The model under review builds one solid part; all positions refer to its coordinate system, in mm. A direction names the side the tool comes from. Round coordinates to 2 decimals unless told otherwise and drop trailing zeros. Write each loop counter-clockwise with the first axis right and the second up, starting at its lowest first coordinate (ties: lowest second). Pieces come first, ordered by that corner, then holes. Notation, with made-up numbers: (-30.75, -19.5) -> (17.25, -19.5) arc R21 cw to (17.25, 18.5) -> close; hole circle Ø1 at (22.5, -30.5). An arc over 180 degrees is marked (long way). Return JSON: item names as keys, results as strings. Group by question number.
1. Clearance check with flat-ended pins moving along their axes: P1, Ø4, axis at y = 2.5, z = -16, coming from the -X side; P2, Ø1.4, axis at x = -58, y = 0.5, coming from the -Z side; P3, Ø4, axis at x = 41, y = 1, coming from the +Z side; P4, Ø6, axis at x = 21.5, z = 11, coming from the -Y side. State where each tip first meets the part, or that it passes through.
2. Take a section at B-B, the plane x = 47. Write out the cut boundary in (y, z).
3. Tool access review of faces 4 (the cylindrical face through (-17.124, 0.049, -11.02)), 5 (the cylindrical face through (-46.17, -0.71, -16.59)), 6 (the cylindrical face through (52.35, -3.25, -2.28)), 7 (the flat face through (-58, 0, 6)), 8 (the flat face through (27, 3, 8)): name each direction out of +Z, -Z, +X, -X, +Y, -Y from which nothing blocks a thin tool from reaching the whole face with its end or side.
4. For line 1 along X through (y, z) = (3.25, 14.5); line 2 along X through (y, z) = (-0.3, 0); line 3 along X through (y, z) = (0.25, -4.5), list the stretches that pass through material, from the lowest coordinate up. Write a range as from..to.
5. Take a section at A-A, the plane x = 3.5. Write out the cut boundary in (y, z).
6. Mouldability with a two-part tool opening along Z and no side actions: class faces 1 (the cylindrical face through (43.01, 1.04, 5.11)), 2 (the cylindrical face through (-54.49, -0.83, 6.51)), 3 (the cylindrical face through (-54.532, -0.827, -6.484)) as pulls with the +Z half, pulls with the -Z half, needs draft (parallel to the pull), parting line crosses it, or undercut.
from build123d import *

# Parameters (mm, degrees)
BOSS_EXTRUDE1_DEPTH = 3.5
CUT_EXTRUDE1_DEPTH  = 65.575537164
SKETCH3_R           = 9.5
CUT_EXTRUDE2_DEPTH  = 5
SKETCH4_R           = 8.75
CUT_EXTRUDE3_DEPTH  = 65.389440128
SKETCH5_R           = 17.5
SKETCH5_R_2         = 10
CUT_EXTRUDE4_DEPTH  = 0.5
SKETCH6_W           = 1.5
SKETCH6_H           = 1.5
FILLET1_START       = 2
FILLET1_DEPTH       = 2
SKETCH7_R           = 6
CUT_EXTRUDE5_DEPTH  = 65.575537164
FILLET2_R           = 3
FILLET3_START       = 2
FILLET3_DEPTH       = 1.5
SKETCH8_R           = 11.25
CUT_EXTRUDE6_DEPTH  = 3
CHAMFER1_SIZE       = 0.5


with BuildPart() as part:
    # Sketch1 → Boss-Extrude1 (new, symmetric)
    with BuildSketch(Plane(origin=(0, 0, 0), x_dir=(1, 0, 0), z_dir=(0, 1, 0))):
        with BuildLine():
            Line((35, -20), (-35, -20))
            ThreePointArc((-35, -20), (-55, 0), (-35, 20))
            Line((-35, 20), (35, 20))
            ThreePointArc((35, 20), (55, 0), (35, -20))
        make_face()
        with BuildLine():
            ThreePointArc((-54.078784028, -6), (-55, 0), (-54.078784028, 6))
            Line((-54.078784028, 6), (-59, 6))
            ThreePointArc((-59, 6), (-60.414213562, 5.414213562), (-61, 4))
            Line((-61, 4), (-61, -4))
            ThreePointArc((-61, -4), (-60.414213562, -5.414213562), (-59, -6))
            Line((-59, -6), (-54.078784028, -6))
        make_face()
    extrude(amount=BOSS_EXTRUDE1_DEPTH, both=True)

    # Sketch2 → Cut-Extrude1 (cut, through all)
    with BuildSketch(Plane(origin=(0, 3.5, 0), x_dir=(1, 0, 0), z_dir=(0, 1, 0))):
        with BuildLine():
            Line((-9, 0.403045012), (-9, 4))
            ThreePointArc((-9, 4), (-9.585786438, 5.414213562), (-11, 6))
            Line((-11, 6), (-14.506098468, 6))
            ThreePointArc((-14.506098468, 6), (-15.634250618, 6.348554352), (-16.369180426, 7.272727273))
            ThreePointArc((-16.369180426, 7.272727273), (-16.754692523, 8.191993351), (-17.185529143, 9.090909091))
            ThreePointArc((-17.185529143, 9.090909091), (-17.109687789, 11.044465936), (-15.404082058, 12))
            Line((-15.404082058, 12), (13.028991175, 12))
            ThreePointArc((13.028991175, 12), (14.979283853, 10.443123537), (13.893211766, 8.196358469))
            Line((13.893211766, 8.196358469), (-6.135779409, -1.400596519))
            ThreePointArc((-6.135779409, -1.400596519), (-8.06572952, -1.289355825), (-9, 0.403045012))
        make_face()
        with BuildLine():
            Line((15.404082058, -12), (-10.197521624, -12))
            ThreePointArc((-10.197521624, -12), (-12.147814303, -10.443123537), (-11.061742215, -8.196358469))
            Line((-11.061742215, -8.196358469), (12.164770585, 2.932699201))
            ThreePointArc((12.164770585, 2.932699201), (14.137811537, 2.793544801), (15.026355614, 1.026416064))
            ThreePointArc((15.026355614, 1.026416064), (15.440463184, -4.174268742), (17.185529143, -9.090909091))
            ThreePointArc((17.185529143, -9.090909091), (17.109687789, -11.044465936), (15.404082058, -12))
        make_face()
    extrude(amount=-CUT_EXTRUDE1_DEPTH, mode=Mode.SUBTRACT)

    # Sketch3 → Cut-Extrude2 (cut)
    with BuildSketch(Plane(origin=(0, 3.5, 0), x_dir=(1, 0, 0), z_dir=(0, 1, 0))):
        with Locations(Location((35, 0, 0), (0, 0, 270))):
            Circle(SKETCH3_R)
    extrude(amount=-CUT_EXTRUDE2_DEPTH, mode=Mode.SUBTRACT)

    # Sketch4 → Cut-Extrude3 (cut, through all)
    with BuildSketch(Plane(origin=(0, -1.5, 0), x_dir=(1, 0, 0), z_dir=(0, 1, 0))):
        with Locations(Location((35, 0, 0), (0, 0, 270))):
            Circle(SKETCH4_R)
    extrude(amount=-CUT_EXTRUDE3_DEPTH, mode=Mode.SUBTRACT)

    # Sketch5 → Cut-Extrude4 (cut)
    with BuildSketch(Plane(origin=(0, 3.5, 0), x_dir=(1, 0, 0), z_dir=(0, 1, 0))):
        with Locations(Location((35, 0, 0), (0, 0, 270))):
            Circle(SKETCH5_R)
        with Locations(Location((35, 0, 0), (0, 0, 270))):
            Circle(SKETCH5_R_2, mode=Mode.SUBTRACT)
    cut_extrude4 = extrude(amount=-CUT_EXTRUDE4_DEPTH, mode=Mode.SUBTRACT)

    # Mirror1: Cut-Extrude4 across plane
    add(cut_extrude4.mirror(Plane.ZX), mode=Mode.SUBTRACT)

    # Sketch6 → Cut-Revolve1 (revolve, cut)
    with BuildSketch(Plane.XY, mode=Mode.PRIVATE) as cut_revolve1_sk:
        with Locations((54.25, 2.75)):
            Rectangle(SKETCH6_W, SKETCH6_H)
    cut_revolve1 = revolve(cut_revolve1_sk.sketch.rotate(Axis((35, -15.42459361, 0), (0, 1, 0)), 90), axis=Axis((35, -15.42459361, 0), (0, 1, 0)), mode=Mode.SUBTRACT)

    # Fillet1: read off the stored shape, not the designer's step
    # Fillet1 outline → Fillet1 (cut)
    with BuildSketch(Plane(origin=(0, 0, 0), x_dir=(1, 0, 0), z_dir=(0, 1, 0)).offset(FILLET1_START)):
        with BuildLine():
            ThreePointArc((35, -20), (30.635642195, -19.518001459), (26.4816458, -18.095238095))
            ThreePointArc((26.4816458, -18.095238095), (27.031628163, -19.21821789), (26.05572809, -20))
            Line((26.05572809, -20), (35, -20))
        make_face()
        with BuildLine():
            ThreePointArc((16.941442804, -11.27926617), (17.755344518, -10.919922264), (18.533450645, -11.351332624))
            ThreePointArc((18.533450645, -11.351332624), (17.82226833, -10.243316586), (17.185529143, -9.090909091))
            ThreePointArc((17.185529143, -9.090909091), (17.391756084, -10.221702427), (16.941442804, -11.27926617))
        make_face()
        with BuildLine():
            ThreePointArc((15.026355614, 1.026416064), (15.13716872, 2.338361293), (15.334061369, 3.640172766))
            ThreePointArc((15.334061369, 3.640172766), (14.799862167, 2.928698763), (13.91017335, 2.924473493))
            ThreePointArc((13.91017335, 2.924473493), (14.752987449, 2.142880559), (15.026355614, 1.026416064))
        make_face()
        with BuildLine():
            ThreePointArc((26.05572809, 20), (27.031628163, 19.21821789), (26.4816458, 18.095238095))
            ThreePointArc((26.4816458, 18.095238095), (30.635642195, 19.518001459), (35, 20))
            Line((35, 20), (26.05572809, 20))
        make_face()
    fillet1 = extrude(amount=FILLET1_DEPTH, mode=Mode.SUBTRACT)

    # Mirror2: Cut-Revolve1, Fillet1 across plane
    add(cut_revolve1.mirror(Plane.ZX), mode=Mode.SUBTRACT)
    add(fillet1.mirror(Plane.ZX), mode=Mode.SUBTRACT)

    # Sketch7 → Cut-Extrude5 (cut, through all)
    with BuildSketch(Plane.XZ.offset(3.5)):
        with Locations(Location((-35, 0, 0), (0, 0, 270))):
            Circle(SKETCH7_R)
    extrude(amount=-CUT_EXTRUDE5_DEPTH, mode=Mode.SUBTRACT)

    # Fillet2
    fillet2_edges = [part.edges().sort_by_distance(p)[0] for p in [
        (-54.078784028, 0, 6),
        (-54.078784028, 0, -6),
    ]]
    fillet(fillet2_edges, radius=FILLET2_R)

    # Mirror3: Cut-Extrude4, Cut-Revolve1 across plane
    add(cut_extrude4.mirror(Plane(origin=(0, 0, 0), x_dir=(0, 0, 1), z_dir=(1, 0, 0))), mode=Mode.SUBTRACT)
    add(cut_revolve1.mirror(Plane(origin=(0, 0, 0), x_dir=(0, 0, 1), z_dir=(1, 0, 0))), mode=Mode.SUBTRACT)

    # Fillet3: read off the stored shape, not the designer's step
    # Fillet3 outline → Fillet3 (cut)
    with BuildSketch(Plane(origin=(0, 0, 0), x_dir=(1, 0, 0), z_dir=(0, 1, 0)).offset(FILLET3_START)):
        with BuildLine():
            ThreePointArc((-53.405226512, -7.826086957), (-53.964760447, -6.351209427), (-54.40631736, -4.836821944))
            ThreePointArc((-54.40631736, -4.836821944), (-54.653584548, -5.769460122), (-55.573977543, -6.058997281))
            ThreePointArc((-55.573977543, -6.058997281), (-54.271017927, -6.67427362), (-53.405226512, -7.826086957))
        make_face()
        with BuildLine():
            ThreePointArc((-55.573977543, 6.058997281), (-54.653584548, 5.769460122), (-54.40631736, 4.836821944))
            ThreePointArc((-54.40631736, 4.836821944), (-53.964760447, 6.351209427), (-53.405226512, 7.826086957))
            ThreePointArc((-53.405226512, 7.826086957), (-54.271017927, 6.67427362), (-55.573977543, 6.058997281))
        make_face()
        with BuildLine():
            Line((-35, -20), (-26.05572809, -20))
            ThreePointArc((-26.05572809, -20), (-27.031628163, -19.21821789), (-26.4816458, -18.095238095))
            ThreePointArc((-26.4816458, -18.095238095), (-30.635642195, -19.518001459), (-35, -20))
        make_face()
        with BuildLine():
            ThreePointArc((-16.369180426, 7.272727273), (-15.93104029, 6.031150433), (-15.575539296, 4.7634364))
            ThreePointArc((-15.575539296, 4.7634364), (-15.380926528, 5.631589563), (-14.571576996, 6.001072147))
            ThreePointArc((-14.571576996, 6.001072147), (-15.661136596, 6.367245602), (-16.369180426, 7.272727273))
        make_face()
        with BuildLine():
            ThreePointArc((-17.185529143, 9.090909091), (-17.391756084, 10.221702427), (-16.941442805, 11.279266171))
            ThreePointArc((-16.941442805, 11.279266171), (-17.755344518, 10.919922264), (-18.533450645, 11.351332624))
            ThreePointArc((-18.533450645, 11.351332624), (-17.82226833, 10.243316586), (-17.185529143, 9.090909091))
        make_face()
        with BuildLine():
            ThreePointArc((-35, 20), (-30.635642195, 19.518001459), (-26.4816458, 18.095238095))
            ThreePointArc((-26.4816458, 18.095238095), (-27.031628163, 19.21821789), (-26.05572809, 20))
            Line((-26.05572809, 20), (-35, 20))
        make_face()
    extrude(amount=FILLET3_DEPTH, mode=Mode.SUBTRACT)

    # Sketch8 → Cut-Extrude6 (cut)
    with BuildSketch(Plane.XZ.offset(3.5)):
        with Locations(Location((-35, 0, 0), (0, 0, 270))):
            Circle(SKETCH8_R)
    extrude(amount=-CUT_EXTRUDE6_DEPTH, mode=Mode.SUBTRACT)

    # Chamfer1
    chamfer1_edges = [part.edges().sort_by_distance(p)[0] for p in [
        (-35, -0.5, 6),
    ]]
    chamfer(chamfer1_edges, length=CHAMFER1_SIZE)


solid = part.part
Output:
{
 "1": {"P1": "stops at x = -49.22", "P2": "stops at z = -6", "P3": "stops at z = 19.6", "P4": "stops at y = -3.5"},
 "2": {"outline": "(-3.5, -14.08) -> (-2, -14.08) -> (-2, -16) -> (2, -16) -> (2, -14.08) -> (3.5, -14.08) -> (3.5, -12.74) -> (3, -12.74) -> (3, 12.74) -> (3.5, 12.74) -> (3.5, 14.08) -> (2, 14.08) -> (2, 16) -> (-2, 16) -> (-2, 14.08) -> (-3.5, 14.08) -> (-3.5, 12.74) -> (-3, 12.74) -> (-3, -12.74) -> (-3.5, -12.74) -> close"},
 "3": {"face 4": "+Y, -Y", "face 5": "-Z, -X, +Y, -Y", "face 6": "-Y", "face 7": "+Z, -X, +Y, -Y", "face 8": "+Y"},
 "4": {"line 1": "x = -46.49..-44.8, -25.2..-23.51, -21.23..21.23, 23.51..25.2, 44.8..46.49", "line 2": "x = -61..-41.3, -28.7..-8.96, -3.21..6.04, 15..25.5, 44.5..55", "line 3": "x = -60.94..-38.97, -31.03..-9.06, 6.18..26.63, 43.37..54.49"},
 "5": {"outline": "(-3.5, -20) -> (3.5, -20) -> (3.5, -12) -> (-3.5, -12) -> close; (-3.5, -3.22) -> (3.5, -3.22) -> (3.5, 1.22) -> (-3.5, 1.22) -> close; (-3.5, 12) -> (3.5, 12) -> (3.5, 20) -> (-3.5, 20) -> close"},
 "6": {"face 1": "undercut", "face 2": "pulls with the +Z half", "face 3": "pulls with the -Z half"}
}
